from build123d import *


with BuildPart() as f1:
    # F0 (on Top) → F1 (revolve)
    with BuildSketch(Plane.XY):
        Polygon((0, 0), (15, 0), (15, 10), (44.5, 10), (45, 10.5), (45, 14.5), (44.5, 15), (0, 15), align=None)
    revolve(axis=Axis((23.765821, 0, 0), (1, 0, 0)))

    # F2: F1 across plane


with BuildPart() as f1_1:
    add(f1.part)
    add(f1.part.mirror(Plane.YZ))


solid = f1_1.part
Build history of the part. All positions in model axes, mm. A direction names the side the tool comes from. Give positions to 0.01 mm unless a question says otherwise; leave off trailing zeros. Loops run counter-clockwise (first coordinate to the right, second up) from the corner with the lowest first, then second, coordinate; pieces in that order, holes last. Notation, with made-up numbers: (83.25, 28.5) - (124.25, 28.5) arc R16 ccw to (124.25, 57.5) - close; hole circle Ø5 at (-20.5, 23). An arc over 180 degrees is marked (long way). Write item = value, one per line. Start each with the question number.
1) Band-saw the part on C-C on x = 34. Give the cut face in (y, z).
2) Drop flat-ended pins along their axis: pin 1 Ø1.5 at (x, y) = (5, 7) entering from -Z; pin 2 Ø3 at (x, z) = (3, -10) entering from +Y; pin 3 Ø10 at (y, z) = (1, 2.5) entering from -X. Give the stop position or say it passes through.
3) Band-saw the part on A-A on z = 0. Give the cut face in (x, y).
4) Tool access for faces 1 (the flat face through (45, -10, 4)), 2 (the cylindrical face through (29.96, -2.17, -9.76)), 3 (the flat face through (-15, 0, 0)): list every direction of +Z, -Z, +X, -X, +Y, -Y with a clear straight run to the whole face (end or side of a thin tool).
5) Pull direction Z, two halves, no side cores. Call faces 4 (the flat face through (15, 0, 0)), 5 (the cylindrical face through (-29.96, -2.17, -9.76)), 6 (the cylindrical face through (0.623, -14.985, 0.66)), 7 (the flat face through (-45, -10, 4)): +Z half, -Z half, draft (parallel to the pull), parting line (faces both ways), or undercut.
6) Band-saw the part on D-D on x = -13. Give the cut face in (y, z).
7) Probe probe 1 along Z at (x, y) = (32.25, 0); probe 2 along Z at (x, y) = (-37, -4); probe 3 along X at (y, z) = (3.5, 8.75). List the from-to ranges inside material, lowest first. Write a range as from..to.
Final values:
q1.outline = circle Ø30 at (0, 0); hole circle Ø20 at (0, 0)
q2.pin_1 = -13.64
q2.pin_2 = 12.36
q2.pin_3 = -15
q3.outline = (-45, -14.5) - (-44.5, -15) - (44.5, -15) - (45, -14.5) - (45, -10.5) - (44.5, -10) - (15, -10) - (15, 10) - (44.5, 10) - (45, 10.5) - (45, 14.5) - (44.5, 15) - (-44.5, 15) - (-45, 14.5) - (-45, 10.5) - (-44.5, 10) - (-15, 10) - (-15, -10) - (-44.5, -10) - (-45, -10.5) - close
q4.face_1 = +Z, -Z, +X, +Y, -Y
q4.face_2 = +X
q4.face_3 = -X
q5.face_4 = undercut
q5.face_5 = undercut
q5.face_6 = parting line
q5.face_7 = draft
q6.outline = circle Ø30 at (0, 0)
q7.probe_1 = -15..-10, 10..15
q7.probe_2 = -14.46..-9.17, 9.17..14.46
q7.probe_3 = -15..15
